from build123d import *

# Parameters (mm, degrees)
SKETCH1_W           = 10
SKETCH1_H           = 10
BOSS_EXTRUDE1_DEPTH = 0.1
CHAMFER1_SIZE       = 0.2
CHAMFER2_SIZE       = 0.5
BOSS_EXTRUDE2_DEPTH = 0.5
BOSS_EXTRUDE2_TAPER = 20
SKETCH3_R           = 0.5
CUT_EXTRUDE1_DEPTH  = 0.01


with BuildPart() as part:
    # Sketch1 → Boss-Extrude1 (new body, symmetric)
    with BuildSketch(Plane(origin=(0, 0, 0), x_dir=(1, 0, 0), z_dir=(0, 1, 0))):
        Rectangle(SKETCH1_W, SKETCH1_H)
    extrude(amount=BOSS_EXTRUDE1_DEPTH, both=True)

    # Chamfer1
    chamfer1_edges = [part.edges().sort_by_distance(p)[0] for p in [
        (5, 0, 5),
        (-5, 0, 5),
        (-5, 0, -5),
    ]]
    chamfer(chamfer1_edges, length=CHAMFER1_SIZE)

    # Chamfer2
    chamfer2_edges = [part.edges().sort_by_distance(p)[0] for p in [
        (5, 0, -5),
    ]]
    chamfer(chamfer2_edges, length=CHAMFER2_SIZE)

    # Sketch2 → Boss-Extrude2 (add)
    with BuildSketch(Plane(origin=(0, 0.1, 0), x_dir=(1, 0, 0), z_dir=(0, 1, 0))):
        Polygon((-4.8, 5), (-5, 4.8), (-5, -4.8), (-4.8, -5), (4.8, -5), (5, -4.8), (5, 4.5), (4.5, 5), align=None)
    boss_extrude2 = extrude(amount=BOSS_EXTRUDE2_DEPTH, taper=BOSS_EXTRUDE2_TAPER)

    # Mirror1: Boss-Extrude2 across plane
    add(boss_extrude2.mirror(Plane.ZX))

    # Sketch3 → Cut-Extrude1 (cut)
    with BuildSketch(Plane(origin=(0, 0.6, 0), x_dir=(1, 0, 0), z_dir=(0, 1, 0))):
        with Locations((4, 4)):
            Circle(SKETCH3_R)
    extrude(amount=-CUT_EXTRUDE1_DEPTH, mode=Mode.SUBTRACT)


solid = part.part
Work out the finished part from the listing and answer in its coordinate system (mm). Round coordinates to 2 decimals unless told otherwise and drop trailing zeros. Answer in a Markdown table with one row per item. Add a question column.
1. Given pin 1 (0.5 mm diameter, centred on x = 4, z = -4, fed in from +Y), flat-ended and moving along its own axis, determine where the tip first touches the part or whether it passes through.
2. The mould has two halves that part along Z. Classify faces 1 (the flat face through (0, 0.6, 0)), 2 (the flat face through (4, 0.59, -4)): +Z half, -Z half, draft (parallel to the pull), parting line (faces both ways), or undercut.
3. Find the intervals of material crossed by line 1 along X through (y, z) = (-0.35, -1); line 2 along Z through (x, y) = (0, -0.2); line 3 along X through (y, z) = (0.55, 4.5), in increasing order. Write a range as from..to.
Worked out:
| question | item | result |
|---|---|---|
| 1 | pin 1 | y = 0.59 |
| 2 | face 1 | draft |
| 2 | face 2 | undercut |
| 3 | line 1 | -4.91..4.91 |
| 3 | line 2 | -4.96..4.96 |
| 3 | line 3 | -4.84..4.84 |
